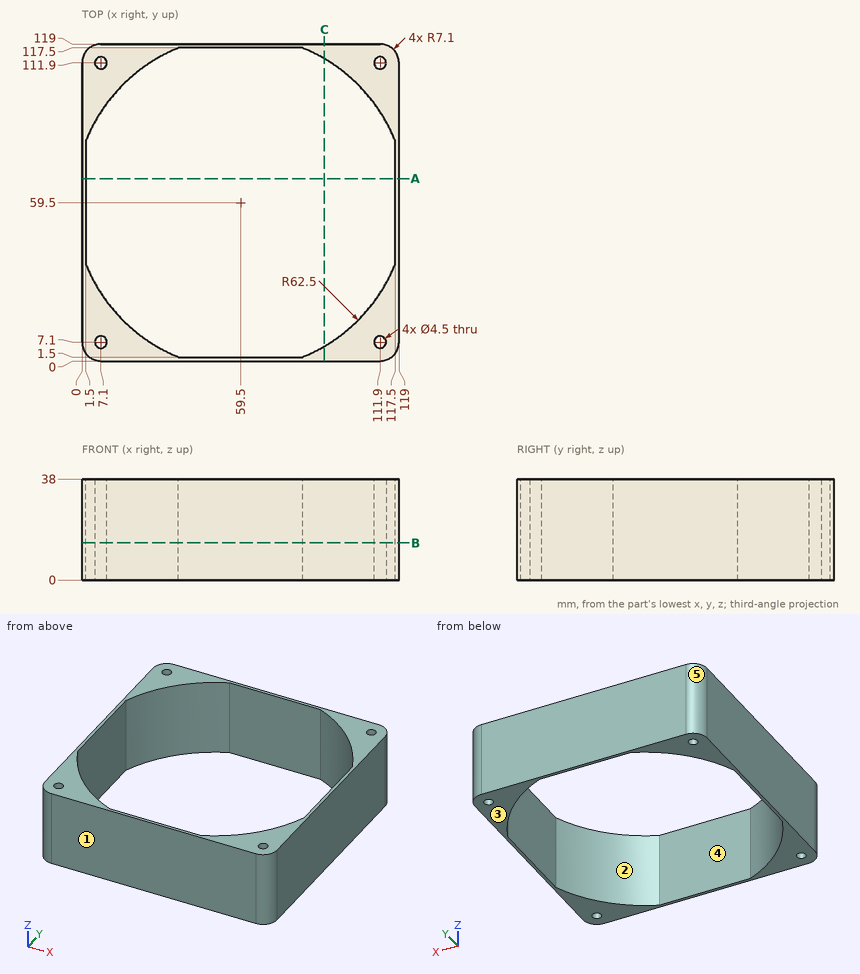
Input: dimensioned drawing with shaded views. Units: mm. Origin: part minimum x, y, z. A direction names the side the tool comes from. Round coordinates to 2 decimals unless told otherwise and drop trailing zeros. Order: outer loops, then holes, each group sorted by start corner. A loop starts at its lowest first (then second) coordinate and runs counter-clockwise, first axis right, second up. Notation, with made-up numbers: (52.5, 60) - (109.5, 60) arc R20 cw to (109.5, 88) - close; hole circle Ø2 at (13.5, 38). An arc over 180 degrees is marked (long way). Answer as a JSON object with one key per item and string values. Group by question number.
(1) Cut plane B-B (z = 14). Return loops of the section in (x, y), then the cut area to 3 significant figures.
(2) Reachability of the marked faces 4 and 5 from +Z, -Z, +X, -X, +Y, -Y: full face, straight path, thin tool, end or side. Return the list, or none.
(3) Pin query (flat end, axial travel): P1, Ø3.5, axis at x = 111.9, y = 7.1, coming from the +Z side. Return the tip coordinate at first contact, or that it passes through.
(4) Material intervals for probe 1 along X at (y, z) = (79.5, 9); probe 2 along Y at (x, z) = (7, 28); probe 3 along X at (y, z) = (110.5, 33), sorted ascending. Write a range as from..to.
(5) Cut plane A-A (y = 68.5). Return loops of the section in (x, z), then the cut area to 3 significant figures.
(6) Draft query along Y for the marked faces 1, 2 and 3. Return one class per face: released by +Y, released by -Y, zero draft, split by the parting line, or undercut.
(7) Cut plane C-C (x = 91). Return loops of the section in (y, z).
Here are the results:
{
 "1": {"outline": "(0, 7.1) arc R7.1 ccw to (7.1, 0) - (111.9, 0) arc R7.1 ccw to (119, 7.1) - (119, 111.9) arc R7.1 ccw to (111.9, 119) - (7.1, 119) arc R7.1 ccw to (0, 111.9) - close; hole (1.5, 36.21) arc R62.5 ccw to (36.21, 1.5) - (82.79, 1.5) arc R62.5 ccw to (117.5, 36.21) - (117.5, 82.79) arc R62.5 ccw to (82.79, 117.5) - (36.21, 117.5) arc R62.5 ccw to (1.5, 82.79) - close; hole circle Ø4.5 at (7.1, 7.1); hole circle Ø4.5 at (7.1, 111.9); hole circle Ø4.5 at (111.9, 7.1); hole circle Ø4.5 at (111.9, 111.9)", "area": "2,350 mm^2"},
 "2": {"face 4": "+Z, -Z", "face 5": "+Z, -Z, -X, +Y"},
 "3": {"P1": "passes through"},
 "4": {"probe 1": "x = 0..1.5, 117.5..119", "probe 2": "y = 0..4.85, 9.35..25.59, 93.41..109.65, 114.15..119", "probe 3": "x = 0..5.34, 8.86..23.37, 95.63..110.14, 113.66..119"},
 "5": {"outline": "(0, 0) - (1.5, 0) - (1.5, 38) - (0, 38) - close; (117.5, 0) - (119, 0) - (119, 38) - (117.5, 38) - close", "area": "114 mm^2"},
 "6": {"face 1": "released by -Y", "face 2": "undercut", "face 3": "zero draft"},
 "7": {"outline": "(0, 0) - (5.52, 0) - (5.52, 38) - (0, 38) - close; (113.48, 0) - (119, 0) - (119, 38) - (113.48, 38) - close"}
}
